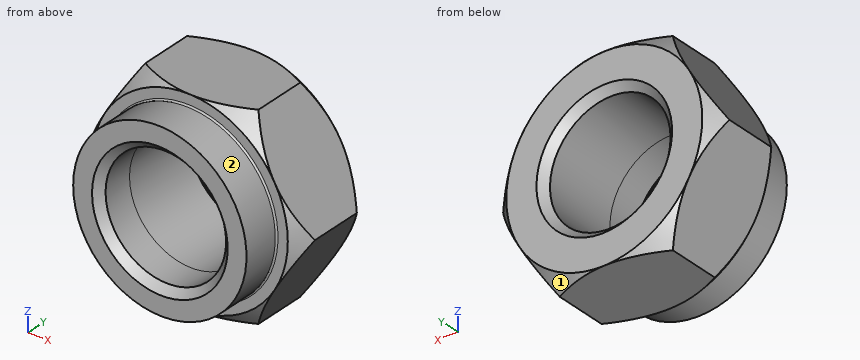
```python
from build123d import *

# Parameters (mm, degrees)
SZKIC1_R                    = 4
DODANIE_WYCI_GNI_CIE1_DEPTH = 5.5
SZKIC2_OUTSIDE_W            = 34.134
SZKIC2_OUTSIDE_H            = 32.122
SZKIC2_OUTSIDE_R            = 6.5
WYTNIJ_WYCI_GNI_CIE29_DEPTH = 6.5
WYTNIJ_WYCI_GNI_CIE29_TAPER = 45
SZKIC4_R                    = 5.75
SZKIC4_R_2                  = 4
DODANIE_WYCI_GNI_CIE2_DEPTH = 2.5
SZKIC5_OUTSIDE_W            = 41.294
SZKIC5_OUTSIDE_H            = 39.282
SZKIC5_OUTSIDE_R            = 6.5
WYTNIJ_WYCI_GNI_CIE30_DEPTH = 10
WYTNIJ_WYCI_GNI_CIE30_TAPER = 45
ZAOKR_GLENIE1_R             = 0.1
SFAZOWANIE1_SIZE            = 0.5


with BuildPart() as part:
    # Szkic1 → Dodanie-wyciągnięcie1 (new body)
    with BuildSketch(Plane(origin=(0, 0, 0), x_dir=(1, 0, 0), z_dir=(0, 1, 0))):
        Polygon((7.505553499, 0), (3.75277675, 6.5), (-3.75277675, 6.5), (-7.505553499, 0), (-3.75277675, -6.5), (3.75277675, -6.5), align=None)
        Circle(SZKIC1_R, mode=Mode.SUBTRACT)
    extrude(amount=DODANIE_WYCI_GNI_CIE1_DEPTH)

    # Szkic2 outside → Wytnij-wyciągnięcie29 (cut, through all)
    with BuildSketch(Plane(origin=(0, 5.5, 0), x_dir=(1, 0, 0), z_dir=(0, 1, 0))):
        Rectangle(SZKIC2_OUTSIDE_W, SZKIC2_OUTSIDE_H)
        Circle(SZKIC2_OUTSIDE_R, mode=Mode.SUBTRACT)
    extrude(amount=-WYTNIJ_WYCI_GNI_CIE29_DEPTH, taper=WYTNIJ_WYCI_GNI_CIE29_TAPER, mode=Mode.SUBTRACT)

    # Szkic4 → Dodanie-wyciągnięcie2 (add)
    with BuildSketch(Plane(origin=(0, 0, 0), x_dir=(-1, 0, 0), z_dir=(0, -1, 0))):
        Circle(SZKIC4_R)
        Circle(SZKIC4_R_2, mode=Mode.SUBTRACT)
    extrude(amount=DODANIE_WYCI_GNI_CIE2_DEPTH)

    # Szkic5 outside → Wytnij-wyciągnięcie30 (cut)
    with BuildSketch(Plane(origin=(0, 0, 0), x_dir=(-1, 0, 0), z_dir=(0, -1, 0))):
        Rectangle(SZKIC5_OUTSIDE_W, SZKIC5_OUTSIDE_H)
        Circle(SZKIC5_OUTSIDE_R, mode=Mode.SUBTRACT)
    extrude(amount=-WYTNIJ_WYCI_GNI_CIE30_DEPTH, taper=WYTNIJ_WYCI_GNI_CIE30_TAPER, mode=Mode.SUBTRACT)

    # Zaokrąglenie1
    zaokr_glenie1_edges = [part.edges().sort_by_distance(p)[0] for p in [
        (5.75, 0, 0),
    ]]
    fillet(zaokr_glenie1_edges, radius=ZAOKR_GLENIE1_R)

    # Sfazowanie1
    sfazowanie1_edges = [part.edges().sort_by_distance(p)[0] for p in [
        (-4, 5.5, 0),
        (4, -2.5, 0),
    ]]
    chamfer(sfazowanie1_edges, length=SFAZOWANIE1_SIZE)


solid = part.part
```
Build history of the part. All positions in model axes, mm. Face numbers are marked on the shaded views. A direction names the side the tool comes from. Round coordinates to 2 decimals unless told otherwise and drop trailing zeros. Write each loop counter-clockwise with the first axis right and the second up, starting at its lowest first coordinate (ties: lowest second). Pieces come first, ordered by that corner, then holes. Notation, with made-up numbers: (62.5, 8.5) -> (100.5, 8.5) arc R20 ccw to (100.5, 34.5) -> close; hole circle Ø10 at (56.5, 11.5). An arc over 180 degrees is marked (long way). Put each result on its own line as item: value.
Item 1: Flat gauge pins, fed straight in: P1, Ø6.5, axis at x = 0, z = 0, coming from the +Y side; P2, Ø3, axis at x = 4, y = -0.5, coming from the +Z side. Where does each tip first touch, or does it go through?
Here are the results:
P1: passes through
P2: stops at z = 6.5
Item 2: Tool access for the marked faces 1 and 2: list every direction of +Z, -Z, +X, -X, +Y, -Y with a clear straight run to the whole face (end or side of a thin tool).
Here are the results:
face 1: -Z, +X, +Y
face 2: -Y
Item 3: Slice it at B-B, the plane y = -1. Give the cut face in (x, z).
Here are the results:
outline: circle Ø11.5 at (0, 0); hole circle Ø8 at (0, 0)
Item 4: Wall check: probe 1 along Z at (x, y) = (0, -1.2); probe 2 along Y at (x, z) = (3.5, 5.25). Give the ranges that are in metal, low to high. Write a range as from..to.
Here are the results:
probe 1: z = -5.75..-4, 4..5.75
probe 2: y = 0..5.5
Item 5: Slice it at A-A, the plane y = 1.5. Give the cut face in (x, z).
Here are the results:
outline: (-7.51, 0) -> (-3.75, -6.5) -> (3.75, -6.5) -> (7.51, 0) -> (3.75, 6.5) -> (-3.75, 6.5) -> close; hole circle Ø8 at (0, 0)
